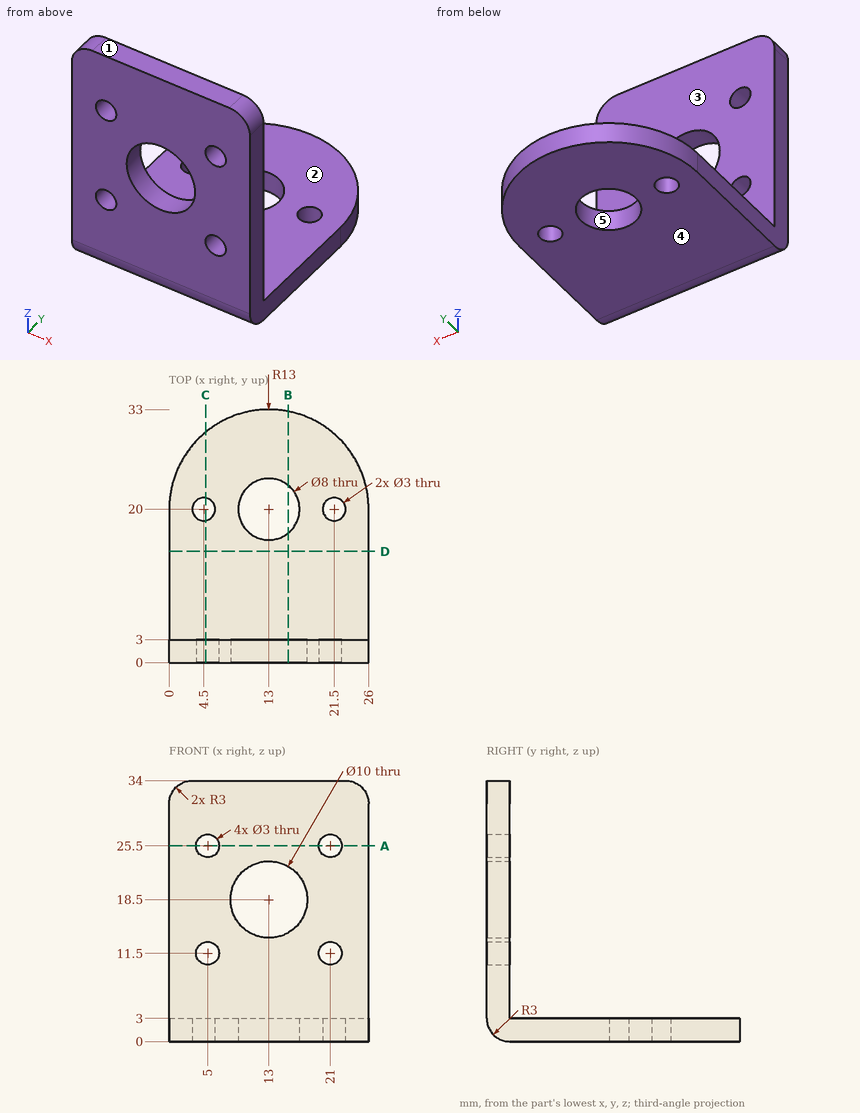
Geometry: see drawing. Coordinates: mm, zero at the bounding-box minimum. A direction names the side the tool comes from. Round coordinates to 2 decimals unless told otherwise and drop trailing zeros. Loops run counter-clockwise (first coordinate to the right, second up) from the corner with the lowest first, then second, coordinate; pieces in that order, holes last. Notation, with made-up numbers: (59, 7) -> (81, 7) arc R27 cw to (81, 37) -> close; hole circle Ø5 at (45.25, -13.75). An arc over 180 degrees is marked (long way). Write each question's results on one line, items separated by ' | '.
Item 1: Cut plane D-D on y = 14.5. Return the cut outline in (x, z), and give its area (3 significant figures).
Answers below:
outline: (0, 0) -> (26, 0) -> (26, 3) -> (0, 3) -> close | area: 78.0 mm²
Item 2: Cut plane A-A on z = 25.5. Return the cut outline in (x, y).
Answers below:
outline: (0, 0) -> (3.5, 0) -> (3.5, 3) -> (0, 3) -> close; (6.5, 0) -> (19.5, 0) -> (19.5, 3) -> (6.5, 3) -> close; (22.5, 0) -> (26, 0) -> (26, 3) -> (22.5, 3) -> close
Item 3: Set-up query: the marked faces 1 and 2. Return all of +Z, -Z, +X, -X, +Y, -Y with unobstructed straight access to the full face (end or side cutting, diameter ignored); none if empty.
Answers below:
face 1: +Z, +X, -X, +Y, -Y | face 2: +Z, +X, -X, +Y
Item 4: Pin query (flat end, axial travel): pin 1 Ø6 at (x, z) = (12, 28.5) entering from +Y; pin 2 Ø1.5 at (x, y) = (22.5, 6.5) entering from +Z. Return the tip coordinate at first contact, or that it passes through.
Answers below:
pin 1: stops at y = 3 | pin 2: stops at z = 3
Item 5: Cut plane B-B on x = 15.5. Return the cut outline in (y, z), and give its area (3 significant figures).
Answers below:
outline: (0, 3) arc R3 ccw to (3, 0) -> (16.88, 0) -> (16.88, 3) -> (3, 3) -> (3, 14.17) -> (0, 14.17) -> close; (0, 22.83) -> (3, 22.83) -> (3, 34) -> (0, 34) -> close; (23.12, 0) -> (32.76, 0) -> (32.76, 3) -> (23.12, 3) -> close | area: 145 mm²
Item 6: Line query: probe 1 along Y at (x, z) = (2.5, 21); probe 2 along Y at (x, z) = (21.5, 1.75). Output: solid intervals per line, ascending. Write a range as [from, to].
Answers below:
probe 1: y = [0, 3] | probe 2: y = [0.27, 18.5], [21.5, 29.84]
Item 7: Cut plane C-C on x = 4.75. Return the cut outline in (y, z).
Answers below:
outline: (0, 3) arc R3 ccw to (3, 0) -> (18.52, 0) -> (18.52, 3) -> (3, 3) -> (3, 10.02) -> (0, 10.02) -> close; (0, 12.98) -> (3, 12.98) -> (3, 24.02) -> (0, 24.02) -> close; (0, 26.98) -> (3, 26.98) -> (3, 34) -> (0, 34) -> close; (21.48, 0) -> (30.05, 0) -> (30.05, 3) -> (21.48, 3) -> close
Item 8: Pull-direction query (Y, two-part tool) for the marked faces 3, 4 and 5; classes: pulls with the +Y half, pulls with the -Y half, needs draft (parallel to the pull), parting line crosses it, or undercut.
Answers below:
face 3: pulls with the +Y half | face 4: needs draft | face 5: undercut
